Source: CAD feature listing. Evaluate the final solid. Frame: model axes, mm. Face numbers are marked on the shaded views. A direction names the side the tool comes from. Give positions to 0.01 mm unless a question says otherwise; leave off trailing zeros. Order: outer loops, then holes, each group sorted by start corner. A loop starts at its lowest first (then second) coordinate and runs counter-clockwise, first axis right, second up. Notation, with made-up numbers: M 77.5,-19 L 125.5,-19 A11 ccw 125.5,-2 Z; hole C 81,-14 d6. An arc over 180 degrees is marked long. Answer as a JSON object with one key per item and string values. Group by question number.
1. Section query C-C (y = -12). Output: boundary loops of the cut face in (x, z), plus the area to 3 significant figures.
2. Set-up query: the marked faces 4, 5 and 6. Return all of +Z, -Z, +X, -X, +Y, -Y with unobstructed straight access to the full face (end or side cutting, diameter ignored); none if empty.
3. Pin query (flat end, axial travel): P1, Ø4, axis at x = 40, y = 19, coming from the +Z side; P2, Ø0.9, axis at x = -14.5, y = -6.5, coming from the +Z side; P3, Ø5, axis at y = -6, z = -39, coming from the +X side. Return the tip coordinate at first contact, or that it passes through.
4. Section query B-B (x = 11.5). Output: boundary loops of the cut face in (y, z).
5. Section query A-A (z = -7.5). Output: boundary loops of the cut face in (x, y), plus the area to 3 significant figures.
6. Material intervals for L1, parallel to Y at x = 18.5, z = -40.5; L2, parallel to Z at x = 20.5, y = -18; L3, parallel to X at y = 10, z = -20.5, sorted ascending. Write a range as [from, to].
7. Section query D-D (x = 38). Output: boundary loops of the cut face in (y, z), plus the area to 3 significant figures.
8. Pull-direction query (X, two-part tool) for the marked faces 1, 2 and 3; classes: +X half, -X half, draft (parallel to the pull), parting line (faces both ways), or undercut.
from build123d import *

# Parameters (mm, degrees)
SKETCH1_W           = 51
SKETCH1_H           = 46
BOSS_EXTRUDE1_DEPTH = 2
SKETCH2_W           = 4
SKETCH2_H           = 46
BOSS_EXTRUDE2_DEPTH = 35
SKETCH3_R           = 1.75
CUT_EXTRUDE1_DEPTH  = 30
SKETCH4_W           = 12
SKETCH4_H           = 46
BOSS_EXTRUDE3_DEPTH = 6
FILLET1_R           = 5
SKETCH5_R           = 2.15
CUT_EXTRUDE2_DEPTH  = 6
SKETCH6_W           = 4
SKETCH6_H           = 7
CUT_EXTRUDE3_DEPTH  = 11
SKETCH7_W           = 4
SKETCH7_H           = 7
CUT_EXTRUDE4_DEPTH  = 11
SKETCH8_R           = 17.5
CUT_EXTRUDE5_DEPTH  = 11
SKETCH9_W           = 13
SKETCH9_H           = 8
BOSS_EXTRUDE4_DEPTH = 25
SKETCH10_R          = 4.5
CUT_EXTRUDE6_DEPTH  = 25
FILLET2_R           = 2


with BuildPart() as part:
    # Sketch1 → Boss-Extrude1 (new body)
    with BuildSketch(Plane.XY):
        Rectangle(SKETCH1_W, SKETCH1_H)
    extrude(amount=BOSS_EXTRUDE1_DEPTH)

    # Sketch2 → Boss-Extrude2 (add)
    with BuildSketch(Plane.XY):
        with Locations((23.5, 0)):
            Rectangle(SKETCH2_W, SKETCH2_H)
        with Locations((-23.5, 0)):
            Rectangle(SKETCH2_W, SKETCH2_H)
    extrude(amount=-BOSS_EXTRUDE2_DEPTH)

    # Sketch3 → Cut-Extrude1 (cut)
    with BuildSketch(Plane(origin=(0, 0, 0), x_dir=(-1, 0, 0), z_dir=(0, 0, -1))):
        with Locations((15.5, -15.5)):
            Circle(SKETCH3_R)
        with Locations((-15.5, -15.5)):
            Circle(SKETCH3_R)
        with Locations((-15.5, 15.5)):
            Circle(SKETCH3_R)
        with Locations((15.5, 15.5)):
            Circle(SKETCH3_R)
    extrude(amount=-CUT_EXTRUDE1_DEPTH, mode=Mode.SUBTRACT)

    # Sketch4 → Boss-Extrude3 (add)
    with BuildSketch(Plane(origin=(0, 0, -35), x_dir=(-1, 0, 0), z_dir=(0, 0, -1))):
        with Locations((-19.5, 0)):
            Rectangle(SKETCH4_W, SKETCH4_H)
        with Locations((19.5, 0)):
            Rectangle(SKETCH4_W, SKETCH4_H)
    extrude(amount=BOSS_EXTRUDE3_DEPTH)

    # Fillet1
    fillet1_edges = [part.edges().sort_by_distance(p)[0] for p in [
        (21.5, 0, -35),
        (-21.5, 0, -35),
    ]]
    fillet(fillet1_edges, radius=FILLET1_R)

    # Sketch5 → Cut-Extrude2 (cut)
    with BuildSketch(Plane(origin=(0, 0, -41), x_dir=(-1, 0, 0), z_dir=(0, 0, -1))):
        with Locations((-18.5, -17)):
            Circle(SKETCH5_R)
        with Locations((-18.5, 17)):
            Circle(SKETCH5_R)
        with Locations((18.5, 17)):
            Circle(SKETCH5_R)
        with Locations((18.5, -17)):
            Circle(SKETCH5_R)
    extrude(amount=-CUT_EXTRUDE2_DEPTH, mode=Mode.SUBTRACT)

    # Sketch6 → Cut-Extrude3 (cut)
    with BuildSketch(Plane(origin=(-13.5, 0, 0), x_dir=(0, 0, -1), z_dir=(1, 0, 0))):
        with Locations((38, 17)):
            Rectangle(SKETCH6_W, SKETCH6_H)
        with Locations((38, -17)):
            Rectangle(SKETCH6_W, SKETCH6_H)
    extrude(amount=-CUT_EXTRUDE3_DEPTH, mode=Mode.SUBTRACT)

    # Sketch7 → Cut-Extrude4 (cut)
    with BuildSketch(Plane.ZY.offset(-13.5)):
        with Locations((-38, -17)):
            Rectangle(SKETCH7_W, SKETCH7_H)
        with Locations((-38, 17)):
            Rectangle(SKETCH7_W, SKETCH7_H)
    extrude(amount=-CUT_EXTRUDE4_DEPTH, mode=Mode.SUBTRACT)

    # Sketch8 → Cut-Extrude5 (cut)
    with BuildSketch(Plane(origin=(0, 0, 0), x_dir=(-1, 0, 0), z_dir=(0, 0, -1))):
        Circle(SKETCH8_R)
    extrude(amount=-CUT_EXTRUDE5_DEPTH, mode=Mode.SUBTRACT)

    # Sketch9 → Boss-Extrude4 (add)
    with BuildSketch(Plane.ZY.offset(-25.5)):
        with Locations((-34.5, 19)):
            Rectangle(SKETCH9_W, SKETCH9_H)
    extrude(amount=-BOSS_EXTRUDE4_DEPTH)

    # Sketch10 → Cut-Extrude6 (cut)
    with BuildSketch(Plane(origin=(50.5, 0, 0), x_dir=(0, 0, -1), z_dir=(1, 0, 0))):
        with Locations((34.5, 15)):
            Circle(SKETCH10_R)
    extrude(amount=-CUT_EXTRUDE6_DEPTH, mode=Mode.SUBTRACT)

    # Fillet2
    fillet2_edges = [part.edges().sort_by_distance(p)[0] for p in [
        (25.5, 19, -28),
        (25.5, 15, -29),
        (25.5, 19.5, -34.5),
        (25.5, 15, -40),
    ]]
    fillet(fillet2_edges, radius=FILLET2_R)


solid = part.part
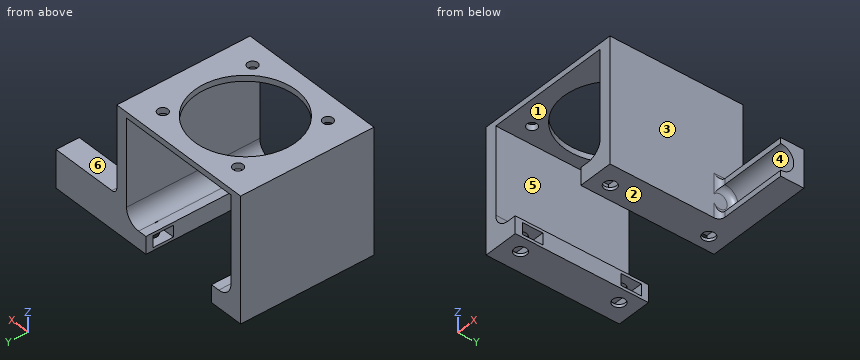
Answer sheet:
{
 "1": {"outline": "M -25.5,-41 L -13.5,-41 L -13.5,-35 L -16.5,-35 A5 cw -21.5,-30 L -21.5,0 L -12.74,0 L -12.74,2 L -25.5,2 Z; M 12.74,0 L 21.5,0 L 21.5,-30 A5 cw 16.5,-35 L 13.5,-35 L 13.5,-41 L 25.5,-41 L 25.5,2 L 12.74,2 Z", "area": "486 mm^2"},
 "2": {"face 4": "+X, -Y", "face 5": "+Y, -Y", "face 6": "+Z, +X, +Y, -Y"},
 "3": {"P1": "z = -28", "P2": "z = -35", "P3": "x = 25.5"},
 "4": {"outline": "M -23,0 L -13.19,0 L -13.19,2 L -23,2 Z; M 13.19,0 L 23,0 L 23,2 L 13.19,2 Z"},
 "5": {"outline": "M -25.5,-23 L -21.5,-23 L -21.5,23 L -25.5,23 Z; M 21.5,-23 L 25.5,-23 L 25.5,23 L 21.5,23 Z", "area": "368 mm^2"},
 "6": {"L1": "[-23, -19.15], [-14.85, 14.85], [19.15, 23]", "L2": "[-41, -40], [-36, -33], [0, 2]", "L3": "[-25.5, -21.5], [21.5, 25.5]"},
 "7": {"outline": "M 15,-41 L 23,-41 L 23,-28 L 15,-28 L 15,-30 A4.5 cw 15,-39 Z", "area": "72.2 mm^2"},
 "8": {"face 1": "undercut", "face 2": "draft", "face 3": "+X half"}
}
